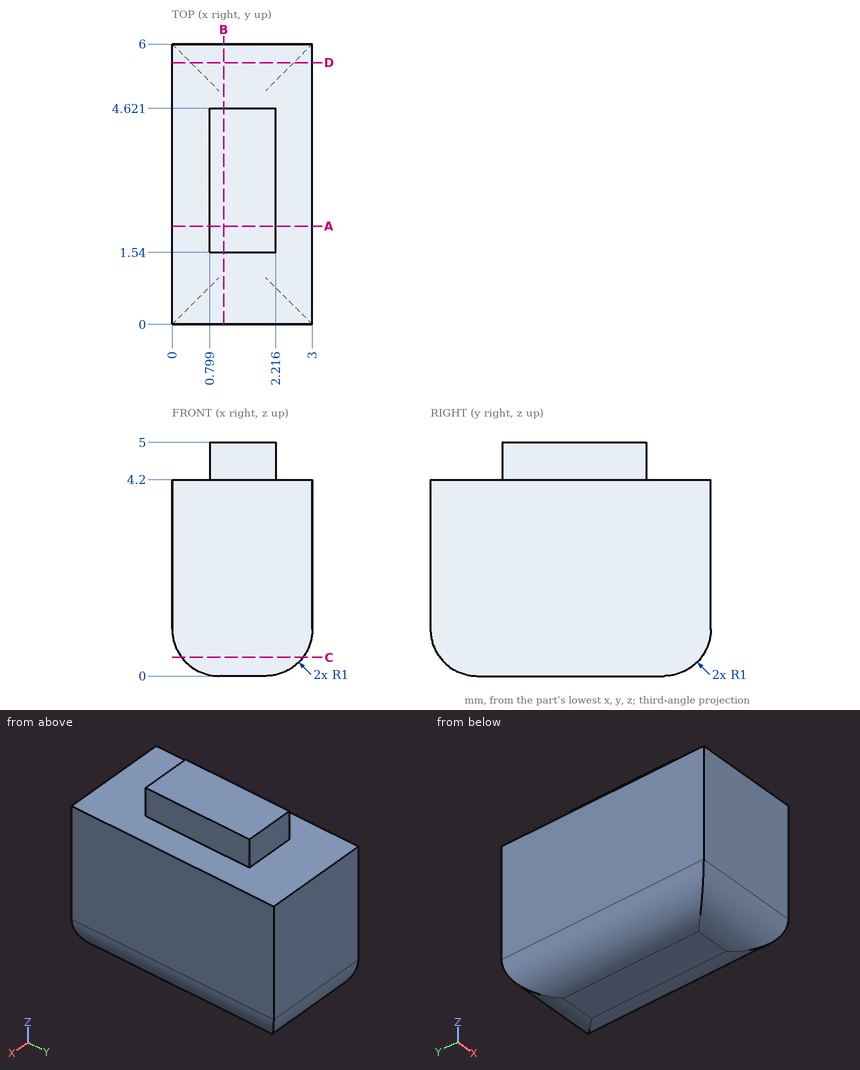
Can you work these out from the drawing? Everything is in mm from the part's minimum corner. Round coordinates to 2 decimals unless told otherwise and drop trailing zeros. Order: outer loops, then holes, each group sorted by start corner. A loop starts at its lowest first (then second) coordinate and runs counter-clockwise, first axis right, second up. Notation, with made-up numbers: M 46,-2.75 L 59,-2.75 A26 ccw 59,33.25 Z; hole C 72.5,-32 d8. An arc over 180 degrees is marked long. One line per question, with ' | ' between items.
1) I need wall thicknesses on line 1 along X through (y, z) = (2.5, 4.65); line 2 along Y through (x, z) = (0.55, 0.8); line 3 along Z through (x, y) = (0.85, 3.5). Which ranges of each line are inside material? Lowest first, please.
Working result:
line 1: 0.8 to 2.22 | line 2: 0.02 to 5.98 | line 3: 0.01 to 5
2) I want a section at D-D, the plane y = 5.6. Write out the boundary of the cut face in (x, z).
Working result:
outline: M 0,1 A1 ccw 0.4,0.2 L 2.6,0.2 A1 ccw 3,1 L 3,4.2 L 0,4.2 Z
3) I want a section at B-B, the plane x = 1.1. Write out the boundary of the cut face in (y, z).
Working result:
outline: M 0,1 A1 ccw 1,0 L 5,0 A1 ccw 6,1 L 6,4.2 L 4.62,4.2 L 4.62,5 L 1.54,5 L 1.54,4.2 L 0,4.2 Z
4) I want a section at C-C, the plane z = 0.4. Write out the boundary of the cut face in (x, y).
Working result:
outline: M 0.2,0.2 L 2.8,0.2 L 2.8,5.8 L 0.2,5.8 Z
5) I want a section at A-A, the plane y = 2.1. Write out the boundary of the cut face in (x, z).
Working result:
outline: M 0,1 A1 ccw 1,0 L 2,0 A1 ccw 3,1 L 3,4.2 L 2.22,4.2 L 2.22,5 L 0.8,5 L 0.8,4.2 L 0,4.2 Z
6) For pin 1 Ø0.6 at (y, z) = (2.5, 5) entering from +X, with a flat end and sliding along its axis, tell me the tip position at first contact or that it passes through.
Working result:
pin 1: x = 2.22
